```python
from build123d import *

# Parameters (mm, degrees)
F0_W     = 15.75
F0_H     = 15.75
F1_DEPTH = 9.55
F2_R     = 2.7655447365
F2_R_2   = 2.8203135122
F3_DEPTH = 2
F4_W     = 12.6326526515
F4_H     = 12.5484350137
F5_DEPTH = 10
F6_W     = 12.4461371452
F6_H     = 12.6247890294
F7_DEPTH = 2.45
F8_R     = 3.25
F8_R_2   = 2.5
F9_DEPTH = 9.58


with BuildPart() as f1:
    # F0 (on Top) → F1 (new body)
    with BuildSketch(Plane.XY):
        with Locations((-2.2300542332, 2.0526186563)):
            Rectangle(F0_W, F0_H)
    extrude(amount=F1_DEPTH)

    # F2 (on Top) → F3 (join)
    with BuildSketch(Plane.XY):
        with BuildLine():
            ThreePointArc((3.3434472608, 8.5381525556), (1.8563335854, 6.422431468), (4.3116325752, 7.2343980162))
            ThreePointArc((4.3116325752, 7.2343980162), (4.3045378825, 7.37322994), (4.2833277224, 7.5106154081))
            ThreePointArc((4.2833277224, 7.5106154081), (3.8683009231, 8.0746128825), (3.3434472608, 8.5381525556))
        make_face()
        with BuildLine():
            ThreePointArc((4.2833277224, 7.5106154081), (4.3045378825, 7.37322994), (4.3116325752, 7.2343980162))
            ThreePointArc((4.3116325752, 7.2343980162), (1.8563335854, 6.422431468), (3.3434472608, 8.5381525556))
            ThreePointArc((3.3434472608, 8.5381525556), (-1.4893392185, 4.3388645246), (4.7318274849, 5.8511244133))
            ThreePointArc((4.7318274849, 5.8511244133), (4.6177266052, 6.7106391599), (4.2833277224, 7.5106154081))
        make_face()
        with BuildLine():
            ThreePointArc((3.3434472608, 8.5381525556), (3.8683009231, 8.0746128825), (4.2833277224, 7.5106154081))
            ThreePointArc((4.2833277224, 7.5106154081), (3.95464834, 8.1535942121), (3.3434472608, 8.5381525556))
        make_face()
        with BuildLine():
            ThreePointArc((-9.0934361556, 7.0864772246), (-6.8414931871, 2.7791078741), (-3.0748776986, 5.8511244133))
            ThreePointArc((-3.0748776986, 5.8511244133), (-4.7421559795, 8.6219651826), (-7.9711833661, 8.4465868163))
            ThreePointArc((-7.9711833661, 8.4465868163), (-8.6298719943, 7.8470325105), (-9.0934361556, 7.0864772246))
        make_face()
        with Locations((-6.210939493, -2.3638040293)):
            Circle(F2_R)
        with Locations((1.4374417951, -2.3638040293)):
            Circle(F2_R_2)
    extrude(amount=-F3_DEPTH)

    # F4 (on Top) → F5 (cut)
    with BuildSketch(Plane.XY):
        with Locations((-2.1983480547, 2.12413189)):
            Rectangle(F4_W, F4_H)
    extrude(amount=F5_DEPTH, mode=Mode.SUBTRACT)

    # F6 (on Top) → F7 (join)
    with BuildSketch(Plane.XY):
        with Locations((-2.1759783849, 2.0920559764)):
            Rectangle(F6_W, F6_H)
    extrude(amount=F7_DEPTH)

    # F8 (on Top) → F9 (join)
    with BuildSketch(Plane.XY):
        with Locations((-2.2931566928, 1.9800718874)):
            Circle(F8_R)
        with Locations((-2.2931566928, 1.9800718874)):
            Circle(F8_R_2, mode=Mode.SUBTRACT)
    extrude(amount=F9_DEPTH)


solid = f1.part
```
CAD build for the part. Positions are in the model's coordinates, mm. A direction names the side the tool comes from. Give positions to 0.01 mm unless a question says otherwise; leave off trailing zeros. Write each loop counter-clockwise with the first axis right and the second up, starting at its lowest first coordinate (ties: lowest second). Pieces come first, ordered by that corner, then holes. Notation, with made-up numbers: M 89,59 L 142,59 A14 cw 142,85 Z; hole C -24.5,-8 d2. An arc over 180 degrees is marked long. Return JSON: item names as keys, results as strings. Group by question number.
(1) Band-saw the part on A-A (z = 8). Give the cut face in (x, y), and give its area (3 significant figures).
(2) Band-saw the part on B-B (y = 1). Give the cut face in (x, z), and give its area (3 significant figures).
(3) Flat gauge pins, fed straight in: pin 1 Ø4 at (x, y) = (-8, -0.5) entering from +Z; pin 2 Ø3 at (x, y) = (-2.29, 1.98) entering from -Z. Where does each tip first touch, or does it go through?
(4) 3-axis set-ups, long thin cutter, end or side, ignore diameter. For faces 1 (the face through (-5.54, 2.12, 5.97)), 2 (the face through (4, 8.1, -1)), 3 (the face through (-8.249, -0.495, -0.986)), 4 (the face through (5.645, 2, 5)): which of +Z, -Z, +X, -X, +Y, -Y reach the whole face in a straight line?
(5) Mould opens along Y. For faces 5 (the face through (-10.105, 2, 5)), 6 (the face through (-2, 9.928, 5)), 7 (the face through (-2, -4.15, 6)), 8 (the face through (4.118, 2, 5)) say: pulls with the +Y half, pulls with the -Y half, needs draft (parallel to the pull), parting line crosses it, or undercut.
(6) Band-saw the part on C-C (x = -2.5). Give the cut face in (y, z), and give its area (3 significant figures).
(7) Band-saw the part on D-D (z = -1). Give the cut face in (x, y), and give its area (3 significant figures).
(8) Drill centre lines: L1, parallel to Y at x = 1.5, z = 5.25; L2, parallel to X at y = -2, z = 3; L3, parallel to Y at x = -0.25, z = 6. Where is each one in solid material? Low to high. Write a range as [from, to].
Entries:
{
 "1": {"outline": "M -10.11,-5.82 L 5.64,-5.82 L 5.64,9.93 L -10.11,9.93 Z; C -2.29,1.98 d6.5; hole M -8.51,-4.15 L 4.12,-4.15 L 4.12,8.4 L -8.51,8.4 Z; hole C -2.29,1.98 d5", "area": "103 mm^2"},
 "2": {"outline": "M -10.11,0 L -8.51,0 L -8.51,9.55 L -10.11,9.55 Z; M -8.4,0 L 4.05,0 L 4.05,2.45 L 0.81,2.45 L 0.81,9.58 L 0.01,9.58 L 0.01,2.45 L -4.59,2.45 L -4.59,9.58 L -5.39,9.58 L -5.39,2.45 L -8.4,2.45 Z; M 4.12,0 L 5.64,0 L 5.64,9.55 L 4.12,9.55 Z", "area": "71.7 mm^2"},
 "3": {"pin 1": "stops at z = 9.55", "pin 2": "stops at z = 0"},
 "4": {"face 1": "+Z", "face 2": "-Z, +X, +Y", "face 3": "-Z", "face 4": "+Z, -Z, +X, +Y, -Y"},
 "5": {"face 5": "needs draft", "face 6": "pulls with the +Y half", "face 7": "undercut", "face 8": "undercut"},
 "6": {"outline": "M -5.82,0 L 9.93,0 L 9.93,9.55 L 8.4,9.55 L 8.4,2.45 L 5.22,2.45 L 5.22,9.58 L 4.47,9.58 L 4.47,2.45 L -0.51,2.45 L -0.51,9.58 L -1.26,9.58 L -1.26,2.45 L -4.15,2.45 L -4.15,9.55 L -5.82,9.55 Z", "area": "72.0 mm^2"},
 "7": {"outline": "C -6.21,5.85 d6.27; C -6.21,-2.36 d5.53; C 1.44,-2.36 d5.64; M 3.34,8.54 A3.29 ccw long 4.28,7.51 A1.36 ccw Z", "area": "114 mm^2"},
 "8": {"L1": "y = [-5.82, -4.15], [8.4, 9.93]", "L2": "x = [-10.11, -8.51], [4.12, 5.64]", "L3": "y = [-5.82, -4.15], [-0.55, 0.54], [3.42, 4.51], [8.4, 9.93]"}
}
